Source: CAD feature listing. Evaluate the final solid. Frame: model axes, mm. A direction names the side the tool comes from. Give positions to 0.01 mm unless a question says otherwise; leave off trailing zeros. Write each loop counter-clockwise with the first axis right and the second up, starting at its lowest first coordinate (ties: lowest second). Pieces come first, ordered by that corner, then holes. Notation, with made-up numbers: (11.25, 11.5) -> (29.25, 11.5) arc R23 cw to (29.25, 26.5) -> close; hole circle Ø5 at (-27, -31). An arc over 180 degrees is marked (long way). Write item = value, one per line.
from build123d import *

# Parameters (mm, degrees)
SKETCH_1_R          = 3.5
EXTRUDE_1_DEPTH     = 4
EXTRUDE_START       = -1.5
EXTRUDE_2_DEPTH     = 1.5
SKETCH_3_R          = 0.5
CUT_EXTRUDE_1_DEPTH = 1.5
SKETCH_4_R          = 1.5
CUT_EXTRUDE_2_DEPTH = 55
SKETCH_5_R          = 2.5
CUT_EXTRUDE_3_DEPTH = 2
CUT_EXTRUDE_START   = -1
SKETCH_6_R          = 2.5
CUT_EXTRUDE_4_DEPTH = 1


with BuildPart() as part:
    # 草图1 → 凸台-拉伸1 (new body)
    with BuildSketch(Plane.XY):
        Circle(SKETCH_1_R)
    extrude(amount=EXTRUDE_1_DEPTH)

    # 草图2 → 凸台-拉伸2 (add)
    with BuildSketch(Plane.XY.offset(4).offset(EXTRUDE_START)):
        with BuildLine():
            Line((0.328125, 3.484585195), (16.1875, 1.99119154))
            ThreePointArc((16.1875, 1.99119154), (18, 0), (16.1875, -1.99119154))
            Line((16.1875, -1.99119154), (0.328125, -3.484585195))
            ThreePointArc((0.328125, -3.484585195), (3.5, 0), (0.328125, 3.484585195))
        make_face()
    extrude(amount=EXTRUDE_2_DEPTH)

    # 草图3 → 切除-拉伸1 (cut)
    with BuildSketch(Plane(origin=(0, 0, 2.5), x_dir=(-1, 0, 0), z_dir=(0, 0, -1))):
        with Locations((-7, 0)):
            Circle(SKETCH_3_R)
        with Locations((-9, 0)):
            Circle(SKETCH_3_R)
        with Locations((-11, 0)):
            Circle(SKETCH_3_R)
        with Locations((-13, 0)):
            Circle(SKETCH_3_R)
        with Locations((-15, 0)):
            Circle(SKETCH_3_R)
        with Locations((-5, 0)):
            Circle(SKETCH_3_R)
        with Locations((-17, 0)):
            Circle(SKETCH_3_R)
    extrude(amount=-CUT_EXTRUDE_1_DEPTH, mode=Mode.SUBTRACT)

    # 草图4 → 切除-拉伸2 (cut)
    with BuildSketch(Plane(origin=(0, 0, 0), x_dir=(-1, 0, 0), z_dir=(0, 0, -1))):
        Circle(SKETCH_4_R)
    extrude(amount=-CUT_EXTRUDE_2_DEPTH, mode=Mode.SUBTRACT)

    # 草图5 → 切除-拉伸3 (cut)
    with BuildSketch(Plane(origin=(0, 0, 0), x_dir=(-1, 0, 0), z_dir=(0, 0, -1))):
        Circle(SKETCH_5_R)
    extrude(amount=-CUT_EXTRUDE_3_DEPTH, mode=Mode.SUBTRACT)

    # 草图6 → 切除-拉伸4 (cut)
    with BuildSketch(Plane.XY.offset(4).offset(CUT_EXTRUDE_START)):
        with Locations(Location((0, 0, 0), (0, 0, 180))):
            Circle(SKETCH_6_R)
    extrude(amount=CUT_EXTRUDE_4_DEPTH, mode=Mode.SUBTRACT)


solid = part.part
1) Material intervals for L1, parallel to Y at x = 5, z = 2.8; L2, parallel to Z at x = 7.25, y = 2; L3, parallel to X at y = -1, z = 0.5, sorted ascending.
Computed:
L1 = -3.04 to -0.5, 0.5 to 3.04
L2 = 2.5 to 4
L3 = -3.35 to -2.29, 2.29 to 3.35
2) Cut plane D-D (x = 8.75). Return the cut outline in (y, z).
Computed:
outline = (-2.69, 2.5) -> (-0.43, 2.5) -> (-0.43, 4) -> (-2.69, 4) -> close; (0.43, 2.5) -> (2.69, 2.5) -> (2.69, 4) -> (0.43, 4) -> close
3) Cut plane C-C (z = 0.85). Return the cut outline in (x, y).
Computed:
outline = circle Ø7 at (0, 0); hole circle Ø5 at (0, 0)
4) Contact query for flat-ended pins moving along their axis: pin 1 (1.5 mm diameter, centred on x = -0.5, y = 1, fed in from +Z); pin 2 (2.5 mm diameter, centred on x = 1, y = -0.5, fed in from -Z). Output: stop coordinate, or through.
Computed:
pin_1 = 3
pin_2 = 2
5) Cut plane B-B (y = -1). Return the cut outline in (x, z).
Computed:
outline = (-3.35, 0) -> (-2.29, 0) -> (-2.29, 2) -> (-1.12, 2) -> (-1.12, 3) -> (-2.29, 3) -> (-2.29, 4) -> (-3.35, 4) -> close; (1.12, 2) -> (2.29, 2) -> (2.29, 0) -> (3.35, 0) -> (3.35, 2.5) -> (17.73, 2.5) -> (17.73, 4) -> (2.29, 4) -> (2.29, 3) -> (1.12, 3) -> close
6) Access query for faces 1 (the flat face through (0, -2, 2)), 2 (the flat face through (0, 2, 3)), 3 (the cylindrical face through (16.523, 0.15, 3.24)). Directions: +Z, -Z, +X, -X, +Y, -Y. A direction counts if a zero-diameter tool reaches every point of the face in a straight line with its end or side. Return the directions, or none.
Computed:
face_1 = -Z
face_2 = +Z
face_3 = +Z, -Z
7) Cut plane A-A (x = 0). Return the cut outline in (y, z).
Computed:
outline = (-3.5, 0) -> (-2.5, 0) -> (-2.5, 2) -> (-1.5, 2) -> (-1.5, 3) -> (-2.5, 3) -> (-2.5, 4) -> (-3.5, 4) -> close; (1.5, 2) -> (2.5, 2) -> (2.5, 0) -> (3.5, 0) -> (3.5, 4) -> (2.5, 4) -> (2.5, 3) -> (1.5, 3) -> close
8) Draft query along X for faces 4 (the flat face through (9, 1, 2.5)), 5 (the flat face through (8.15, 2.75, 3.24)), 6 (the cylindrical face through (0.54, -2.44, 0.99)). Return one class per face: pulls with the +X half, pulls with the -X half, needs draft (parallel to the pull), parting line crosses it, or undercut.
Computed:
face_4 = needs draft
face_5 = pulls with the +X half
face_6 = undercut
